Geometry: final body of the model. Coordinates: model frame, mm. A direction names the side the tool comes from. Round coordinates to 2 decimals unless told otherwise and drop trailing zeros. Write each loop counter-clockwise with the first axis right and the second up, starting at its lowest first coordinate (ties: lowest second). Pieces come first, ordered by that corner, then holes. Notation, with made-up numbers: (17, 45.5) -> (76, 45.5) arc R20 ccw to (76, 67.5) -> close; hole circle Ø10 at (0, -33.75). An arc over 180 degrees is marked (long way). One line per item, written item: value. Start each with the question number.
from build123d import *

# Parameters (mm, degrees)
CROQUIS1_R              = 7.75
SALIENTE_EXTRUIR1_DEPTH = 27
CROQUIS2_W              = 6.5
CROQUIS2_H              = 6.5
CORTAR_EXTRUIR1_DEPTH   = 30.139749484
CROQUIS3_R              = 5
SALIENTE_EXTRUIR2_DEPTH = 5
CROQUIS4_R              = 1.75
CORTAR_EXTRUIR2_DEPTH   = 30.139749484
CROQUIS5_R              = 3.25
CORTAR_EXTRUIR3_DEPTH   = 10


with BuildPart() as part:
    # Croquis1 → Saliente-Extruir1 (new body)
    with BuildSketch(Plane.XY):
        Circle(CROQUIS1_R)
    extrude(amount=-SALIENTE_EXTRUIR1_DEPTH)

    # Croquis2 → Cortar-Extruir1 (cut, through all)
    with BuildSketch(Plane.XY):
        Rectangle(CROQUIS2_W, CROQUIS2_H)
    extrude(amount=-CORTAR_EXTRUIR1_DEPTH, mode=Mode.SUBTRACT)

    # Croquis3 → Saliente-Extruir2 (add)
    with BuildSketch(Plane(origin=(0, 0, -27), x_dir=(-1, 0, 0), z_dir=(0, 0, -1))):
        Circle(CROQUIS3_R)
    extrude(amount=-SALIENTE_EXTRUIR2_DEPTH)

    # Croquis4 → Cortar-Extruir2 (cut, through all)
    with BuildSketch(Plane(origin=(0, 0, -27), x_dir=(-1, 0, 0), z_dir=(0, 0, -1))):
        Circle(CROQUIS4_R)
    extrude(amount=-CORTAR_EXTRUIR2_DEPTH, mode=Mode.SUBTRACT)

    # Croquis5 → Cortar-Extruir3 (cut)
    with BuildSketch(Plane(origin=(0, 0, -27), x_dir=(-1, 0, 0), z_dir=(0, 0, -1))):
        Circle(CROQUIS5_R)
    extrude(amount=-CORTAR_EXTRUIR3_DEPTH, mode=Mode.SUBTRACT)


solid = part.part
(1) Line query: probe 1 along Y at (x, z) = (0, -24.7); probe 2 along Z at (x, y) = (2.75, -2); probe 3 along Y at (x, z) = (-3, -20.5). Output: solid intervals per line, ascending.
(2) Section query A-A (z = -16). Output: boundary loops of the cut face in (x, y), and give its area (3 significant figures).
(3) Set-up query: faces 5 (the face through (-3.25, 0, -11)), 6 (the face through (-4, 0, 0)). Return all of +Z, -Z, +X, -X, +Y, -Y with unobstructed straight access to the full face (end or side cutting, diameter ignored); none if empty.
(4) Section query D-D (x = -5.25). Output: boundary loops of the cut face in (y, z).
(5) Pin query (flat end, axial travel): pin 1 (2 mm diameter, centred on y = 1.5, z = -8, fed in from -X); pin 2 (1 mm diameter, centred on x = -2.5, y = -1, fed in from +Z); pin 3 (8 mm diameter, centred on x = -4.5, z = -15, fed in from +Y). Return the tip coordinate at first contact, or that it passes through.
(6) Pull-direction query (X, two-part tool) for faces 1 (the face through (-1.009, 7.684, -13.311)), 2 (the face through (2, -3, -27)), 3 (the face through (3.25, 0, -11)), 4 (the face through (0, -3.25, -11)); classes: pulls with the +X half, pulls with the -X half, needs draft (parallel to the pull), parting line crosses it, or undercut.
(7) Section query C-C (x = 0.75). Output: boundary loops of the cut face in (y, z), and give its area (3 significant figures).
(8) Section query B-B (y = 2.25). Output: boundary loops of the cut face in (x, z).
Results list:
1. probe 1: y = -7.75 to -3.25, 3.25 to 7.75
1. probe 2: z = -27 to -22
1. probe 3: y = -7.15 to -3.25, 3.25 to 7.15
2. outline: circle Ø15.5 at (0, 0); hole (-3.25, -3.25) -> (3.25, -3.25) -> (3.25, 3.25) -> (-3.25, 3.25) -> close
2. area: 146 mm^2
3. face 5: +Z
3. face 6: +Z, +X, -X, +Y, -Y
4. outline: (-5.7, -27) -> (5.7, -27) -> (5.7, 0) -> (-5.7, 0) -> close
5. pin 1: stops at x = -7.73
5. pin 2: passes through
5. pin 3: stops at y = 7.73
6. face 1: parting line crosses it
6. face 2: needs draft
6. face 3: undercut
6. face 4: undercut
7. outline: (-7.71, -27) -> (-3.16, -27) -> (-3.16, -22) -> (-3.25, -22) -> (-3.25, 0) -> (-7.71, 0) -> close; (3.16, -27) -> (7.71, -27) -> (7.71, 0) -> (3.25, 0) -> (3.25, -22) -> (3.16, -22) -> close
7. area: 242 mm^2
8. outline: (-7.42, -27) -> (-2.35, -27) -> (-2.35, -22) -> (-3.25, -22) -> (-3.25, 0) -> (-7.42, 0) -> close; (2.35, -27) -> (7.42, -27) -> (7.42, 0) -> (3.25, 0) -> (3.25, -22) -> (2.35, -22) -> close
